from build123d import *

# Parameters (mm, degrees)
F1_DEPTH      = 1.5
F2_W          = 71
F2_H          = 5.37
F3_DEPTH      = 1
F5_DEPTH      = 1.5
F6_R          = 2.125
F7_DEPTH      = 25
F7_DEPTH_BACK = 25
F8_W          = 6.5
F8_H          = 18
F9_DEPTH      = 3.5
F10_R         = 1


with BuildPart() as f1:
    # F0 (on Front) → F1 (new body)
    with BuildSketch(Plane.XZ):
        Polygon((0, 50), (0, 0), (35, 0), (75, 40), (75, 50), align=None)
    extrude(amount=F1_DEPTH)

    # F2 (on face) → F3 (join)
    with BuildSketch(Plane(origin=(0, 0, 0), x_dir=(-1, 0, 0), z_dir=(0, 1, 0))):
        Polygon((0, 0), (0, 50), (-75, 50), (-75, 40), (-35, 0), align=None)
        Polygon((-2, 7.63), (-2, 2), (-34.1715728753, 2), (-39.8015728753, 7.63), align=None, mode=Mode.SUBTRACT)
        Polygon((-44.8015728753, 12.63), (-66.4248850161, 34.2533121408), (-7.7811020593, 12.63), align=None, mode=Mode.SUBTRACT)
        Polygon((-2, 14.7616253496), (-64.020470816, 37.63), (-2, 37.63), align=None, mode=Mode.SUBTRACT)
        with Locations((-37.5, 45.315)):
            Rectangle(F2_W, F2_H, mode=Mode.SUBTRACT)
    extrude(amount=F3_DEPTH)

    # F4 (on face) → F5 (join)
    with BuildSketch(Plane(origin=(0, 1, 0), x_dir=(-1, 0, 0), z_dir=(0, 1, 0))):
        Polygon((0, 0), (0, 50), (-75, 50), (-75, 40), (-35, 0), align=None)
    extrude(amount=F5_DEPTH)

    # F6 (on face) → F7 (cut, two sides)
    with BuildSketch(Plane(origin=(0, 0, 0), x_dir=(-1, 0, 0), z_dir=(0, 1, 0))) as f7_sk:
        with Locations((-9.84, 40.13)):
            Circle(F6_R)
        with Locations((-9.84, 10.13)):
            Circle(F6_R)
        with Locations((-30.32, 40.13)):
            Circle(F6_R)
        with Locations((-30.32, 10.13)):
            Circle(F6_R)
        with Locations((-50, 40.13)):
            Circle(F6_R)
        with Locations((-65, 40.13)):
            Circle(F6_R)
    extrude(amount=-F7_DEPTH, mode=Mode.SUBTRACT)
    extrude(f7_sk.sketch, amount=F7_DEPTH_BACK, mode=Mode.SUBTRACT)

    # F8 (on face) → F9 (join)
    with BuildSketch(Plane(origin=(0, 2.5, 0), x_dir=(-1, 0, 0), z_dir=(0, 1, 0))):
        with Locations((-9.84, 25.13)):
            Rectangle(F8_W, F8_H)
        with Locations((-30.32, 25.13)):
            Rectangle(F8_W, F8_H)
    extrude(amount=F9_DEPTH)

    # F10
    f10_edges = [f1.edges().sort_by_distance(p)[0] for p in [
        (33.57, 6, 25.13),
        (27.07, 6, 25.13),
        (13.09, 6, 25.13),
        (6.59, 6, 25.13),
        (0, 0.5, 50),
        (0, 0.5, 0),
        (75, 0.5, 50),
        (75, 0.5, 40),
        (35, 0.5, 0),
    ]]
    fillet(f10_edges, radius=F10_R)


solid = f1.part
The listing builds one solid part. Answer for the finished solid, in the listing's coordinates (mm). A direction names the side the tool comes from. Round coordinates to 2 decimals unless told otherwise and drop trailing zeros. Write each loop counter-clockwise with the first axis right and the second up, starting at its lowest first coordinate (ties: lowest second). Pieces come first, ordered by that corner, then holes. Notation, with made-up numbers: (-30.75, 48.5) - (-2.75, 48.5) arc R22 cw to (-2.75, 63.5) - close; hole circle Ø5 at (77.25, 43.5). An arc over 180 degrees is marked (long way). Use a Markdown table: item, result. Add a question column.
1. For a pull along X with two mould halves and no side action, classify faces 5 (the face through (33.57, 4, 25)), 6 (the face through (37, 0, 50)), 7 (the face through (38, 1, 45)) as +X half, -X half, draft (parallel to the pull), parting line (faces both ways), or undercut.
2. The part is cut by section A-A (z = 10.13). Write down the section's boundary in (x, y) (3 decimals), and give its area (3 significant figures).
3. The part is cut by section B-B (z = 45.5). Write down the section's boundary in (x, y).
4. Flat-ended cylindrical pins translate along their axes: P1, Ø2.5, axis at x = 30.32, z = 10.13, coming from the -Y side; P2, Ø1.1, axis at y = 0.5, z = 24, coming from the +X side; P3, Ø2, axis at y = -0.5, z = 34, coming from the +X side; P4, Ø0.8, axis at y = 3.5, z = 29, coming from the +X side. Find the tip coordinate at first contact, or state that the pin passes through.
5. Consider line 1 (Z direction, x = 65, y = 0.85) (3 decimals); line 2 (Y direction, x = 41, z = 31); line 3 (X direction, y = 2.25, z = 9.5). Determine where each line is inside the solid, lowest interval first.
6. The part is cut by section C-C (x = 65). Write down the section's boundary in (y, z) (3 decimals).
7. The part is cut by section D-D (x = 9.84). Give the number of separate pieces and of enclosed holes in the cut face, and give its area (3 significant figures).
8. A tool of negligible diameter and unlimited length cuts with its end or side. For faces 1 (the face through (27.07, 4, 25)), 2 (the face through (10, 4, 16.13)), 3 (the face through (30, 4, 34.13)), 4 (the face through (39, 0, 20)), from which of +Z, -Z, +X, -X, +Y, -Y can it reach the whole face along a straight path? Write none if from no direction.
Reported:
| question | item | result |
|---|---|---|
| 1 | face 5 | +X half |
| 1 | face 6 | draft |
| 1 | face 7 | undercut |
| 2 | outline | (0, -1.5) - (7.715, -1.5) - (7.715, 2.5) - (0, 2.5) - close; (11.965, -1.5) - (28.195, -1.5) - (28.195, 2.5) - (11.965, 2.5) - close; (32.445, -1.5) - (45.13, -1.5) - (45.13, 2.5) - (32.445, 2.5) - close |
| 2 | area | 147 mm^2 |
| 3 | outline | (0, -1.5) - (75, -1.5) - (75, 2.5) - (0, 2.5) - close; hole (2, 0) - (73, 0) - (73, 1) - (2, 1) - close |
| 4 | P1 | through |
| 4 | P2 | x = 59.55 |
| 4 | P3 | x = 70 |
| 4 | P4 | x = 33.57 |
| 5 | line 1 | 30 to 32.828, 33.728 to 38.005, 42.255 to 42.63, 48 to 50 |
| 5 | line 2 | -1.5 to 0, 1 to 2.5 |
| 5 | line 3 | 0 to 7.81, 11.87 to 28.29, 32.35 to 44.5 |
| 6 | outline | (-1.5, 30) - (2.5, 30) - (2.5, 38.005) - (-1.5, 38.005) - close; (-1.5, 42.255) - (2.5, 42.255) - (2.5, 50) - (-1.5, 50) - close; hole (0, 32.828) - (1, 32.828) - (1, 33.728) - (0, 33.728) - close; hole (0, 42.63) - (1, 42.63) - (1, 48) - (0, 48) - close |
| 7 | separate pieces | 3 |
| 7 | enclosed holes | 4 |
| 7 | area | 197 mm^2 |
| 8 | face 1 | +Z, -Z, +Y |
| 8 | face 2 | -Z, +X, -X, +Y |
| 8 | face 3 | +Z, +X, -X, +Y |
| 8 | face 4 | none |
